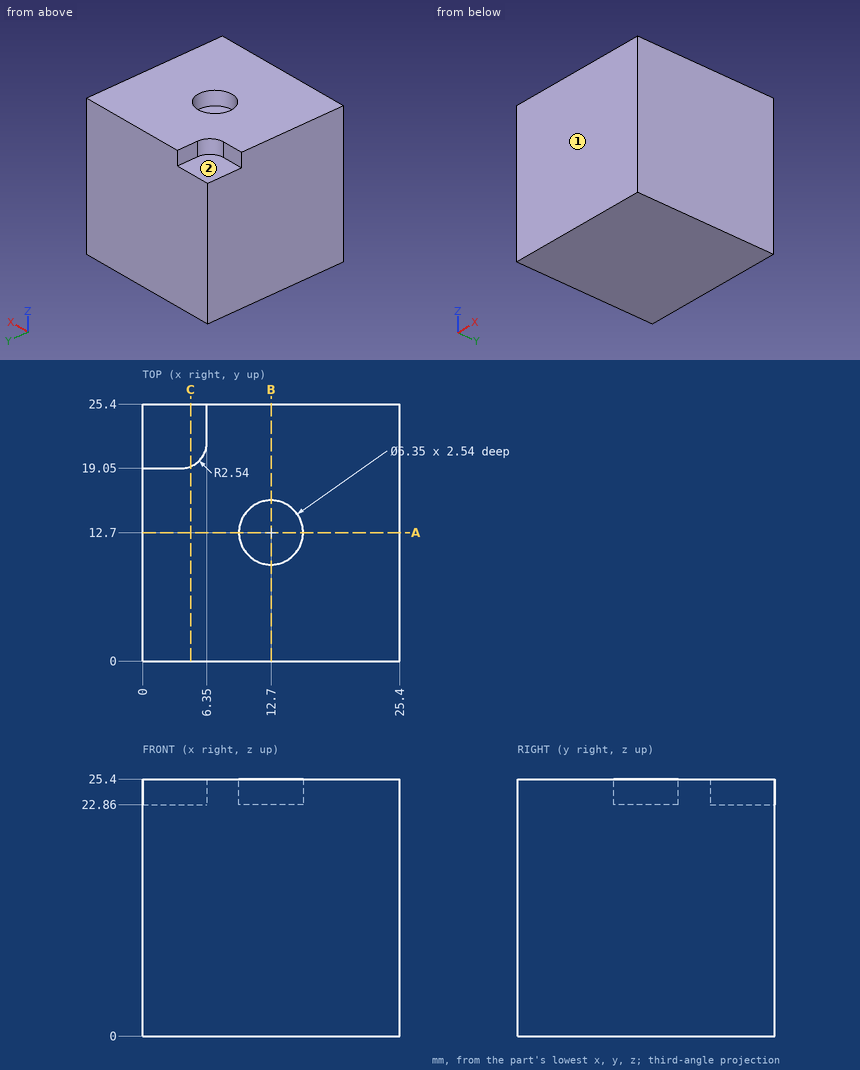
Drawing for the job (mm, zero at the part's lowest x, y, z). A direction names the side the tool comes from. Round coordinates to 2 decimals unless told otherwise and drop trailing zeros. Write each loop counter-clockwise with the first axis right and the second up, starting at its lowest first coordinate (ties: lowest second). Pieces come first, ordered by that corner, then holes. Notation, with made-up numbers: M 23.5,-6.5 L 81.5,-6.5 A23 ccw 81.5,28.5 Z; hole C 60,26 d4. An arc over 180 degrees is marked long. Answer as a JSON object with one key per item and string values. Group by question number.
(1) Drill centre lines: L1, parallel to Y at x = 12.7, z = 24.4 (3 decimals); L2, parallel to Z at x = 11.5, y = 15. Where is each one in solid material? Low to high.
(2) Flat gauge pins, fed straight in: pin 1 (1.9 mm diameter, centred on x = 4, y = 21, fed in from +Z); pin 2 (2 mm diameter, centred on x = 2.5, z = 24.5, fed in from +Y); pin 3 (0.8 mm diameter, centred on y = 23, z = 23.5, fed in from -X). Where does each tip first touch, or does it go through?
(3) Cut at C-C (x = 4.75). Give the cut face in (y, z).
(4) Cut at A-A (y = 12.7). Give the cut face in (x, z) (3 decimals).
(5) Which spindle directions (+Z, -Z, +X, -X, +Y, -Y) get a long thin tool onto all of the face, cutting with end or side? Do the marked faces 1 and 2. Say none if no direction does.
Responses:
{
 "1": {"L1": "y = 0 to 9.525, 15.875 to 25.4", "L2": "z = 0 to 22.86"},
 "2": {"pin 1": "stops at z = 22.86", "pin 2": "stops at y = 19.05", "pin 3": "stops at x = 6.35"},
 "3": {"outline": "M 0,0 L 25.4,0 L 25.4,22.86 L 19.23,22.86 L 19.23,25.4 L 0,25.4 Z"},
 "4": {"outline": "M 0,0 L 25.4,0 L 25.4,25.4 L 15.875,25.4 L 15.875,22.86 L 9.525,22.86 L 9.525,25.4 L 0,25.4 Z"},
 "5": {"face 1": "+Z, -Z, +X, -X, -Y", "face 2": "+Z, -X, +Y"}
}
